The listing builds one solid part. Answer for the finished solid, in the listing's coordinates (mm). Face numbers are marked on the shaded views. A direction names the side the tool comes from. Round coordinates to 2 decimals unless told otherwise and drop trailing zeros. Loops run counter-clockwise (first coordinate to the right, second up) from the corner with the lowest first, then second, coordinate; pieces in that order, holes last. Notation, with made-up numbers: M 44.5,68 L 80.5,68 A15 cw 80.5,82 Z; hole C 18,27.25 d2. An arc over 180 degrees is marked long. Answer as a JSON object with one key per item and string values.
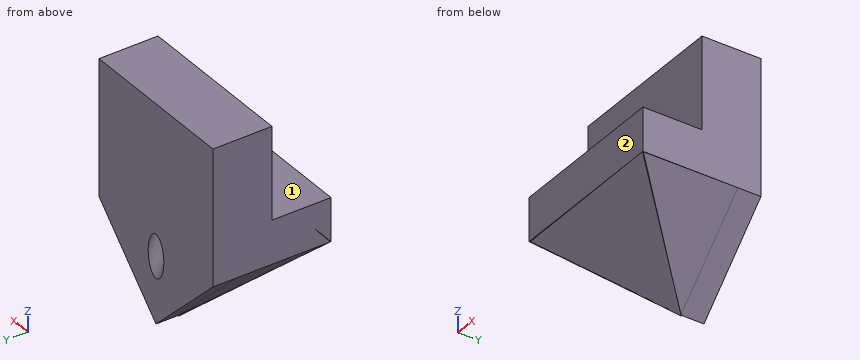
```python
from build123d import *

# Parameters (mm, degrees)
F0_W      = 45.0838953257
F0_H      = 11.9667137042
F1_DEPTH  = 32.47426
F3_DEPTH  = 6.35
F4_W      = 45.0838953257
F4_H      = 16.23713
F5_DEPTH  = 25.4
F7_DEPTH  = 15.33327
F9_DEPTH  = 15.1057
F12_DEPTH = 6.35
F15_R     = 3.0971764623
F16_DEPTH = 50.8


with BuildPart() as f1:
    # F0 (on Front) → F1 (new body)
    with BuildSketch(Plane.XZ):
        Rectangle(F0_W, F0_H)
    extrude(amount=F1_DEPTH)

    # F2 (on face) → F3 (join)
    with BuildSketch(Plane(origin=(0, 0, 0), x_dir=(-1, 0, 0), z_dir=(0, 1, 0))):
        Polygon((-22.5419476628, -5.9833568521), (0, -28.2688885927), (22.5419476628, -5.9833568521), align=None)
    extrude(amount=-F3_DEPTH)

    # F4 (on face) → F5 (join)
    with BuildSketch(Plane.XY.offset(5.9833568521)):
        with Locations((0, -8.118565)):
            Rectangle(F4_W, F4_H)
    extrude(amount=F5_DEPTH)

    # F6 (on face) → F7 (join)
    with BuildSketch(Plane(origin=(-14.1335193941, 0, -14.2961387765), x_dir=(0.7111398414, 0, -0.7030505857), z_dir=(-0.7030505857, 0, -0.7111398414))):
        Polygon((-11.8238745458, 6.35), (19.8744586816, 6.35), (-11.7087624967, 32.2476960719), align=None)
    extrude(amount=-F7_DEPTH)

    # F8 (on face) → F9 (join)
    with BuildSketch(Plane(origin=(14.1335193941, 0, -14.2961387765), x_dir=(0.7111398414, 0, 0.7030505857), z_dir=(0.7030505857, 0, -0.7111398414))):
        Polygon((11.742355302, 32.341375947), (-19.8744586816, 6.35), (11.8238745458, 6.35), align=None)
    extrude(amount=-F9_DEPTH)

    # F11 (on 3pt) → F12 (join)
    with BuildSketch(Plane(origin=(-0.0840004707, -16.6552165824, -19.4391446065), x_dir=(0.999994616, -0.0021350351, -0.0024919073), z_dir=(0.0032814596, 0.6506323042, 0.7593858287))):
        Polygon((22.4465951324, -20.7644402981), (0, 13.771279715), (-22.5187186152, -20.7644402981), align=None)
    extrude(amount=F12_DEPTH)

    # F15 (on 3pt) → F16 (cut)
    with BuildSketch(Plane(origin=(0, -18.3562553404, 30.0906216504), x_dir=(1, 0, 0), z_dir=(0, 0.5207793852, -0.8536912978))):
        with Locations((0, 5.1728854887)):
            Circle(F15_R)
    extrude(amount=F16_DEPTH, mode=Mode.SUBTRACT)


solid = f1.part
```
Item 1: The part is cut by section B-B (z = -17). Give the vertices of the cut face in (x, y) (3 decimals), then the cut area to 3 significant figures.
Values follow:
{"outline": "M -11.479,-19.445 L -11.399,-19.445 L -11.399,-19.493 L -11.317,-19.445 L 11.332,-19.56 L 11.282,-19.458 L 11.399,-19.527 L 11.399,0 L -11.399,0 L -11.399,-19.282 Z", "area": "445 mm^2"}
Item 2: Straight lines are drawn through the part: line 1 (X direction, y = -7.5, z = 16); line 2 (X direction, y = -15, z = 15); line 3 (Y direction, x = 5, z = 20.5). For each, find the intervals that lie inside material, in ascending order.
Values follow:
{"line 1": "-22.54 to 22.54", "line 2": "-22.54 to -3.09, 3.09 to 22.54", "line 3": "-16.24 to 0"}
Item 3: The part is cut by section A-A (x = 2). Give the number of separate pieces and of enclosed holes in the cut face, then the cut area to 3 significant figures.
Values follow:
{"separate pieces": "2", "enclosed holes": "1", "area": "1,070 mm^2"}
Item 4: Which of the six approach directions +Z, -Z, +X, -X, +Y, -Y give full straight-line access (tool end or side, diameter ignored) to the marked faces 1 and 2?
Values follow:
{"face 1": "+Z, +X, -X, -Y", "face 2": "+Z, -Z, +X, -X, -Y"}
Item 5: Flat-ended cylindrical pins translate along their axes: P1, Ø10, axis at x = -12, z = -15, coming from the +Y side; P2, Ø3.5, axis at x = 0.5, y = -15, coming from the -Z side; P3, Ø5, axis at x = -6.5, y = -25, coming from the +Z side; P4, Ø16, axis at y = -23.5, z = 22, coming from the -X side. Find the tip coordinate at first contact, or state that the pin passes through.
Values follow:
{"P1": "y = 0", "P2": "z = -22.36", "P3": "z = 5.98", "P4": "x = -22.54"}
